Autodesk Inventor part; units mm, degrees
ref_plane "YZ Plane" through (0, 0, 0) normal (1, 0, 0) x (0, 1, 0)
ref_plane "XZ Plane" through (0, 0, 0) normal (0, 1, 0) x (-1, 0, 0)
ref_plane "XY Plane" through (0, 0, 0) normal (0, 0, 1) x (1, 0, 0)
sketch "Skizze1" plane through (0, 0, 0) normal (0, 0, 1) x (1, 0, 0)
  line L0 (0, 0) -> (95, 0)
  line L1 (95, 0) -> (95, 120)
  line L2 (95, 120) -> (0, 120)
  line L3 (0, 120) -> (0, 0)
  circle A0 centre (38.1, 37.9782) radius 2.905
  circle A1 centre (90, 42.5) radius 1.5
  circle A2 centre (24.7598, 24.638) radius 2.905
  circle A3 centre (38.1, 11.2978) radius 2.905
  circle A4 centre (51.4402, 24.638) radius 2.905
  circle A5 centre (90, 92.5) radius 1.5
  circle A6 centre (25, 42.5) radius 1.5
  circle A7 centre (25, 92.5) radius 1.5
  line L4 (0, 120) -> (240, 120)
  line L5 (240, 120) -> (240, 0)
  line L6 (240, 0) -> (0, 0)
  line L7 (0, 0) -> (0, 120)
  circle A8 centre (222, 112) radius 1.5
  circle A9 centre (122, 112) radius 1.5
  circle A10 centre (222, 47) radius 1.5
  circle A11 centre (122, 47) radius 1.5
  point P0 (38.1, 24.638)
  dimension "d0" = 120
  dimension "d1" = 95
  dimension "d5" = 5
  dimension "d6" = 3
  dimension "d12" = 360
  dimension "d16" = 50
  dimension "d19" = 65
  dimension "d69" = 42.5
  dimension "d99" = 240
  dimension "d100" = 120
  dimension "d103" = 8
  dimension "d104" = 18
  dimension "d105" = 3
  dimension "d108" = 100
  dimension "d111" = 65
  dimension "d114" = 47
extrude "Extrusion2" add sketch "Skizze1" against normal blind 10 contours L3 L2 L1 L0 | L1 L4 L5 L6 | A0 | A2 | A3 | A4 | A8 | A9 | A10 | A11
hole "Bohrung8" at (122, 112, 0) at (222, 112, 0) at (222, 47, 0) at (122, 47, 0) direction (0, 0, -1) diameter 2.459 depth 9 tip angle 118
sketch "Skizze11" plane through (0, 0, -10) normal (0, 0, -1) x (-1, 0, 0)
  circle A0 centre (-25, 92.5) radius 1.5
  circle A1 centre (-25, 42.5) radius 1.5
  circle A2 centre (-90, 92.5) radius 1.5
  circle A3 centre (-90, 42.5) radius 1.5
hole "Bohrung11" at (25, 42.5, -10) at (90, 42.5, -10) at (90, 92.5, -10) at (25, 92.5, -10) direction (0, 0, 1) diameter 4.3 depth 13 tip angle 118 counterbore diameter 7.5 counterbore depth 4.5
sketch "Skizze12" plane through (0, 0, 0) normal (0, 0, 1) x (1, 0, 0)
  circle A0 centre (25, 92.5) radius 2.15
  circle A1 centre (25, 42.5) radius 2.15
  line L0 (240, 120) -> (0, 120)
  line L1 (25, 92.5) -> (25, 42.5)
  circle A2 centre (25, 82.5) radius 1.5
  circle A3 centre (25, 52.5) radius 1.5
  circle A4 centre (90, 82.5) radius 1.5
  circle A5 centre (90, 52.5) radius 1.5
  dimension "d163" = 3
  dimension "d164" = 10
  dimension "d167" = 30
  dimension "d170" = 65
hole "Bohrung12" at (25, 82.5, 0) at (25, 52.5, 0) at (90, 52.5, 0) at (90, 82.5, 0) direction (0, 0, -1) diameter 3 depth 8 tip angle 118
fillet "Rundung1" radius 4 4 edges at (240, 0, -5) (0, 0, -5) (0, 120, -5) (240, 120, -5)
equation "\"d100\" = d0"
properties part number "Paddle_Base"
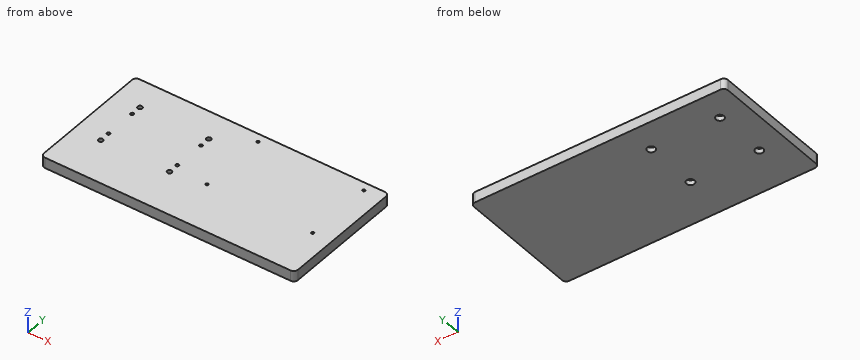
Build history of the part. All positions in model axes, mm. Give positions to 0.01 mm unless a question says otherwise; leave off trailing zeros. Loops run counter-clockwise (first coordinate to the right, second up) from the corner with the lowest first, then second, coordinate; pieces in that order, holes last.
Item 1: Drill centre lines: line 1 (Y direction, x = 25, z = -7.05); line 2 (X direction, y = 52.5, z = -3.25); line 3 (Y direction, x = 25, z = -2.6). Where is each one in solid material? Low to high.
Answers follow:
line 1: y = 0 to 38.75, 46.25 to 51, 54 to 81, 84 to 88.75, 96.25 to 120
line 2: x = 0 to 23.5, 26.5 to 88.5, 91.5 to 240
line 3: y = 0 to 40.35, 44.65 to 51, 54 to 81, 84 to 90.35, 94.65 to 120
Item 2: Flat gauge pins, fed straight in: pin 1 (5.5 mm diameter, centred on x = 90, y = 42.5, fed in from -Z); pin 2 (2.5 mm diameter, centred on x = 90, y = 52.5, fed in from +Z). Where does each tip first touch, or does it go through?
Answers follow:
pin 1: stops at z = -5.5
pin 2: stops at z = -8.15
Item 3: Slice it at A-A, the plane y = 42.5. List the corners of the cut face in (x, z), and give its area (3 significant figures).
Answers follow:
outline: (0, -10) - (21.25, -10) - (21.25, -5.5) - (22.85, -5.5) - (22.85, 0) - (0, 0) - close; (27.15, -5.5) - (28.75, -5.5) - (28.75, -10) - (86.25, -10) - (86.25, -5.5) - (87.85, -5.5) - (87.85, 0) - (27.15, 0) - close; (92.15, -5.5) - (93.75, -5.5) - (93.75, -10) - (240, -10) - (240, 0) - (92.15, 0) - close
area: 2,290 mm2
